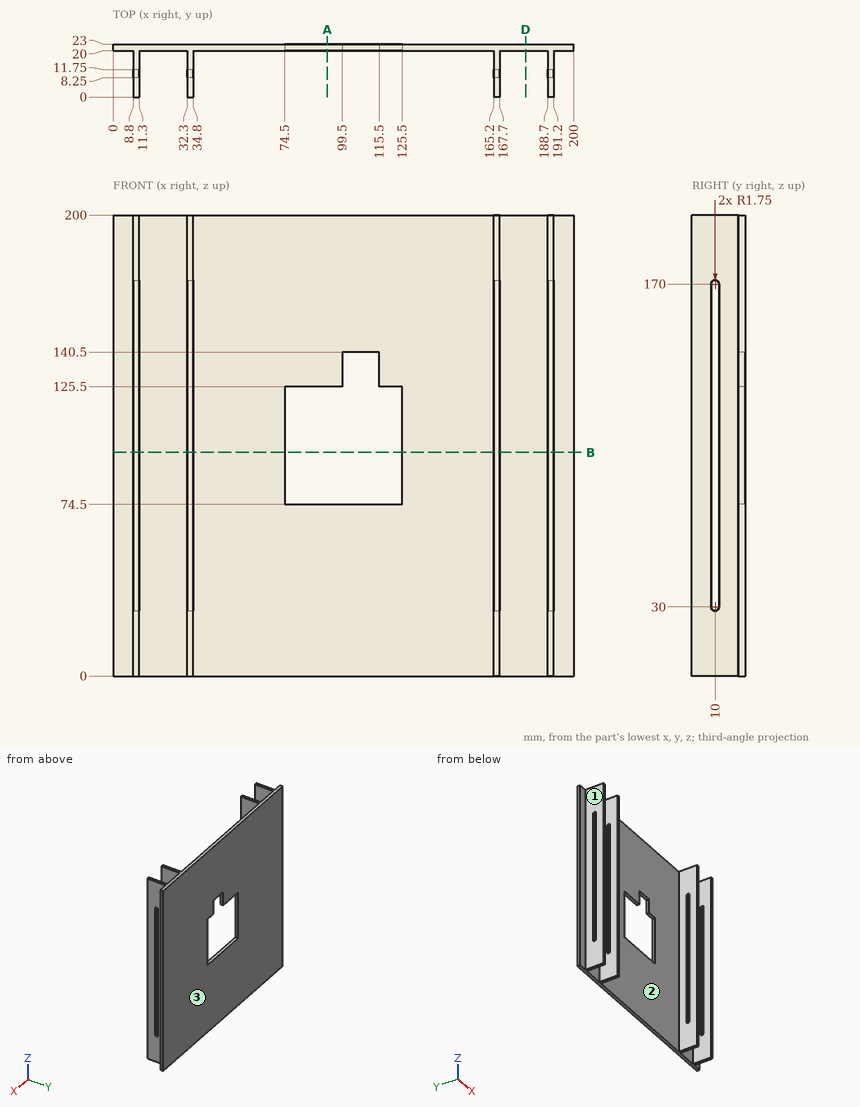
Answer from the drawing. Dimensions are ordinates in mm from the lowest x, y and z of the part. Give positions to 0.01 mm unless a question says otherwise; leave off trailing zeros. Write each loop counter-clockwise with the first axis right and the second up, starting at its lowest first coordinate (ties: lowest second). Pieces come first, ordered by that corner, then holes. Notation, with made-up numbers: (31.25, 13.5) - (44.25, 13.5) arc R11 ccw to (44.25, 24.5) - close; hole circle Ø5 at (-2, 41.5). An arc over 180 degrees is marked (long way). Answer in a Markdown table with one row per item. Add a question column.
Item 1: Section B-B, the plane z = 97 is taken. Count the separate pieces of the cut face and the enclosed holes in it, and give its area (3 significant figures).
Item 2: Determine the mould class of the marked faces 1, 2 and 3 for opening direction X: pulls with the +X half, pulls with the -X half, needs draft (parallel to the pull), parting line crosses it, or undercut.
Item 3: Flat-ended cylindrical pins translate along their axes: P1, Ø10, axis at x = 78.5, z = 23.5, coming from the -Y side; P2, Ø10, axis at y = 5, z = 98, coming from the +X side; P3, Ø6, axis at y = 14, z = 107.5, coming from the -X side. Find the tip coordinate at first contact, or state that the pin passes through.
Item 4: Section D-D, the plane x = 179 is taken. Write down the section's boundary in (y, z), and give its area (3 significant figures).
Item 5: Find the intervals of material crossed by L1, parallel to X at y = 12.5, z = 10; L2, parallel to Y at x = 9, z = 120.5; L3, parallel to Y at x = 88.5, z = 151.5, in increasing order.
Item 6: Section A-A, the plane x = 93 is taken. Write down the section's boundary in (y, z), and give its area (3 significant figures).
Recorded:
| question | item | result |
|---|---|---|
| 1 | separate pieces | 6 |
| 1 | enclosed holes | 0 |
| 1 | area | 612 mm2 |
| 2 | face 1 | pulls with the -X half |
| 2 | face 2 | undercut |
| 2 | face 3 | needs draft |
| 3 | P1 | stops at y = 20 |
| 3 | P2 | stops at x = 191.2 |
| 3 | P3 | stops at x = 8.8 |
| 4 | outline | (20, 0) - (23, 0) - (23, 200) - (20, 200) - close |
| 4 | area | 600 mm2 |
| 5 | L1 | x = 8.8 to 11.3, 32.3 to 34.8, 165.2 to 167.7, 188.7 to 191.2 |
| 5 | L2 | y = 0 to 8.25, 11.75 to 23 |
| 5 | L3 | y = 20 to 23 |
| 6 | outline | (20, 0) - (23, 0) - (23, 74.5) - (20, 74.5) - close; (20, 125.5) - (23, 125.5) - (23, 200) - (20, 200) - close |
| 6 | area | 447 mm2 |
